```python
from build123d import *

# Parameters (mm, degrees)
F0_R     = 22.704104
F1_DEPTH = 609.6
F3_D     = 41.91
F4_R     = 21.826729
F5_DEPTH = 457.2


with BuildPart() as f1:
    # F0 (on Right) → F1 (new body)
    with BuildSketch(Plane.YZ):
        Circle(F0_R)
    extrude(amount=F1_DEPTH)

    # F3 (through all)
    with Locations(Plane(origin=(0, 0, 0), x_dir=(0, -1, 0), z_dir=(-1, 0, 0))):
        with Locations((0, 0)):
            Hole(F3_D / 2)

    # F4 (on Front) → F5 (join)
    with BuildSketch(Plane.XZ):
        with Locations((44.85634, 0)):
            Circle(F4_R)
    extrude(amount=F5_DEPTH)


solid = f1.part
```
Geometry check sheet. Reference: the model listing, model coordinates, mm. A direction names the side the tool comes from. Round coordinates to 2 decimals unless told otherwise and drop trailing zeros. Order: outer loops, then holes, each group sorted by start corner. A loop starts at its lowest first (then second) coordinate and runs counter-clockwise, first axis right, second up. Notation, with made-up numbers: (-7.75, -3.5) - (9.25, -3.5) arc R14 ccw to (9.25, 17.5) - close; hole circle Ø10 at (8.25, 25). An arc over 180 degrees is marked (long way). Use a Markdown table: item, result. Add a question column.
1) Gauge pin test, flat ends, axial feed: P1, Ø8, axis at x = 452.5, z = 18, coming from the -Y side; P2, Ø6, axis at y = -190, z = -0.5, coming from the +X side; P3, Ø8, axis at y = -87.5, z = -10, coming from the +X side. Record the tip position at first contact, or that the pin passes through.
2) Thickness scan on line 1 along Y through (x, z) = (286, 0) (3 decimals); line 2 along Y through (x, z) = (401, 14). Record the ranges inside material, lowest first.
3) Section check C-C (y = -244). Record the cut outline in (x, z), then the cut area to 3 significant figures.
4) Mould release check, pull along Z, two halves, no side actions. Record for faces 4 (the flat face through (45, -457.2, 0)), 5 (the cylindrical face through (300.533, 21.656, 6.82)), 6 (the cylindrical face through (23.033, -8.002, 0.393)): released by +Z, released by -Z, zero draft, split by the parting line, or undercut.
5) Set-up check for faces 1 (the cylindrical face through (23.05, -228.57, 0.96)), 2 (the flat face through (0, 7, -20)), 3 (the flat face through (45, 0, 0)): record each of +Z, -Z, +X, -X, +Y, -Y from which the full face is reachable in a straight line by a thin tool's end or side.
6) Section check A-A (z = 0). Record the cut outline in (x, y) (3 decimals), then the cut area to 3 significant figures.
7) Section check B-B (x = 572). Record the cut outline in (y, z) (3 decimals), then the cut area to 3 significant figures.
Established:
| question | item | result |
|---|---|---|
| 1 | P1 | y = -17.87 |
| 1 | P2 | x = 66.68 |
| 1 | P3 | x = 65.84 |
| 2 | line 1 | -22.704 to -20.955, 20.955 to 22.704 |
| 2 | line 2 | -17.87 to -15.59, 15.59 to 17.87 |
| 3 | outline | circle Ø43.65 at (44.86, 0) |
| 3 | area | 1,500 mm2 |
| 4 | face 4 | zero draft |
| 4 | face 5 | split by the parting line |
| 4 | face 6 | undercut |
| 5 | face 1 | -Y |
| 5 | face 2 | +Z, -Z, -X, +Y, -Y |
| 5 | face 3 | +X, -X |
| 6 | outline | (0, -22.704) - (23.03, -22.704) - (23.03, -457.2) - (66.683, -457.2) - (66.683, -22.704) - (609.6, -22.704) - (609.6, -20.955) - (66.683, -20.955) - (66.683, 0) - (23.03, 0) - (23.03, -20.955) - (0, -20.955) - close; (0, 20.955) - (609.6, 20.955) - (609.6, 22.704) - (0, 22.704) - close |
| 6 | area | 22,000 mm2 |
| 7 | outline | circle Ø45.408 at (0, 0); hole circle Ø41.91 at (0, 0) |
| 7 | area | 240 mm2 |
